Check sheet for the modelled part. Datum: model origin and axes. Units: mm. A direction names the side the tool comes from. Round coordinates to 2 decimals unless told otherwise and drop trailing zeros. Order: outer loops, then holes, each group sorted by start corner. A loop starts at its lowest first (then second) coordinate and runs counter-clockwise, first axis right, second up. Notation, with made-up numbers: (-12, 17) -> (36, 17) arc R23 ccw to (36, 46) -> close; hole circle Ø9 at (47, -9.5). An arc over 180 degrees is marked (long way). Answer in a Markdown table with one row per item. Add a question column.
1. Sectioned sample at D-D, the plane z = -23. Record the boundary of the cut face in (x, y).
2. Sectioned sample at A-A, the plane y = 0. Record the boundary of the cut face in (x, z).
3. Sectioned sample at C-C, the plane z = -2.5. Record the boundary of the cut face in (x, y), then the cut area to 3 significant figures.
4. Access from +Z, -Z, +X, -X, +Y, -Y to the whole of each face (thin tool, end or side, straight path). Record for faces 1 (the flat face through (0, 0, 0)), 2 (the flat face through (0, 1, -4)), 3 (the cylindrical face through (-0.108, 0.488, -24.257)).
5. Depth check by flat-ended pin: P1, Ø1, axis at y = -0.5, z = -33.5, coming from the -X side; P2, Ø1.5, axis at x = 0, z = -6, coming from the +Y side; P3, Ø0.6, axis at x = 0, y = 1, coming from the +Z side; P4, Ø1, axis at x = 0.5, z = -35, coming from the +Y side. Enter the tip coordinate at first touch or a pass-through.
6. Sectioned sample at B-B, the plane x = 0. Record the boundary of the cut face in (y, z).
7. Material ranges on L1, parallel to Z at x = 1.1, y = 0.7; L2, parallel to X at y = -0.1, z = -6.5; L3, parallel to Y at x = 0.3, z = -18, recorded low to high. Write a range as from..to.
```python
from build123d import *

# Parameters (mm, degrees)
SKETCH1_R           = 1.5
BOSS_EXTRUDE1_DEPTH = 9.27
CUT_EXTRUDE1_DEPTH  = 8.67
SKETCH3_R           = 0.5
BOSS_EXTRUDE2_DEPTH = 30.5
FILLET1_R           = 0.1


with BuildPart() as part:
    # Sketch1 → Boss-Extrude1 (new body)
    with BuildSketch(Plane.XY):
        Circle(SKETCH1_R)
    extrude(amount=-BOSS_EXTRUDE1_DEPTH)

    # Sketch2 → Cut-Extrude1 (cut)
    with BuildSketch(Plane.XY):
        with BuildLine():
            Line((-1.118033989, 1), (1.118033989, 1))
            ThreePointArc((1.118033989, 1), (0, 1.5), (-1.118033989, 1))
        make_face()
    extrude(amount=-CUT_EXTRUDE1_DEPTH, mode=Mode.SUBTRACT)

    # Sketch3 → Boss-Extrude2 (add)
    with BuildSketch(Plane(origin=(0, 0, -9.27), x_dir=(-1, 0, 0), z_dir=(0, 0, -1))):
        with Locations(Location((0, 0, 0), (0, 0, 180))):
            Circle(SKETCH3_R)
    extrude(amount=BOSS_EXTRUDE2_DEPTH)

    # Fillet1
    fillet1_edges = [part.edges().sort_by_distance(p)[0] for p in [
        (-0.5, 0, -39.77),
        (-0.535233135, -1.401258538, 0),
    ]]
    fillet(fillet1_edges, radius=FILLET1_R)


solid = part.part
```
Answer key:
| question | item | result |
|---|---|---|
| 1 | outline | circle Ø1 at (0, 0) |
| 2 | outline | (-1.5, -9.27) -> (-0.5, -9.27) -> (-0.5, -39.67) arc R0.1 ccw to (-0.4, -39.77) -> (0.4, -39.77) arc R0.1 ccw to (0.5, -39.67) -> (0.5, -9.27) -> (1.5, -9.27) -> (1.5, -0.1) arc R0.1 ccw to (1.4, 0) -> (-1.4, 0) arc R0.1 ccw to (-1.5, -0.1) -> close |
| 3 | outline | (-1.12, 1) arc R1.5 ccw (long way) to (1.12, 1) -> close |
| 3 | area | 6.29 mm² |
| 4 | face 1 | +Z, +X, -X, +Y, -Y |
| 4 | face 2 | +Z, +X, -X, +Y |
| 4 | face 3 | -Z |
| 5 | P1 | stops at x = -0.5 |
| 5 | P2 | stops at y = 1 |
| 5 | P3 | stops at z = 0 |
| 5 | P4 | stops at y = 0.5 |
| 6 | outline | (-1.5, -9.27) -> (-0.5, -9.27) -> (-0.5, -39.67) arc R0.1 ccw to (-0.4, -39.77) -> (0.4, -39.77) arc R0.1 ccw to (0.5, -39.67) -> (0.5, -9.27) -> (1.5, -9.27) -> (1.5, -8.67) -> (1, -8.67) -> (1, 0) -> (-1.4, 0) arc R0.1 ccw to (-1.5, -0.1) -> close |
| 7 | L1 | z = -9.27..0 |
| 7 | L2 | x = -1.5..1.5 |
| 7 | L3 | y = -0.4..0.4 |
